Part model, mm, in its own coordinate system. Round coordinates to 2 decimals unless told otherwise and drop trailing zeros. Loops run counter-clockwise (first coordinate to the right, second up) from the corner with the lowest first, then second, coordinate; pieces in that order, holes last. Notation, with made-up numbers: (50, 82.5) -> (77, 82.5) arc R16 ccw to (77, 97.5) -> close; hole circle Ø1 at (31, 54.25). An arc over 180 degrees is marked (long way). Use a Markdown table: item, result. Add a question column.
Item 1: Cut at D-D, the plane x = -18. List the corners of the cut face in (y, z).
Item 2: Flat gauge pins, fed straight in: pin 1 (1.2 mm diameter, centred on y = 4.5, z = 1.5, fed in from -X); pin 2 (0.7 mm diameter, centred on y = 31, z = 1, fed in from -X); pin 3 (1.2 mm diameter, centred on x = -16.5, z = 1.5, fed in from -Y). Where does each tip first touch, or does it go through?
Item 3: Cut at B-B, the plane z = 1.8. List the corners of the cut face in (x, y).
Item 4: Cut at A-A, the plane x = -11.65. List the corners of the cut face in (y, z), plus the area to 3 significant figures.
Item 5: Probe line 1 (Y direction, x = -14.75, z = 0.55); line 2 (Y direction, x = -12.25, z = 1.5); line 3 (X direction, y = 31, z = 2.05). List the from-to ranges inside material, lowest first. Write a range as [from, to].
Item 6: Cut at C-C, the plane y = 50.5. List the corners of the cut face in (x, z), plus the area to 4 significant figures.
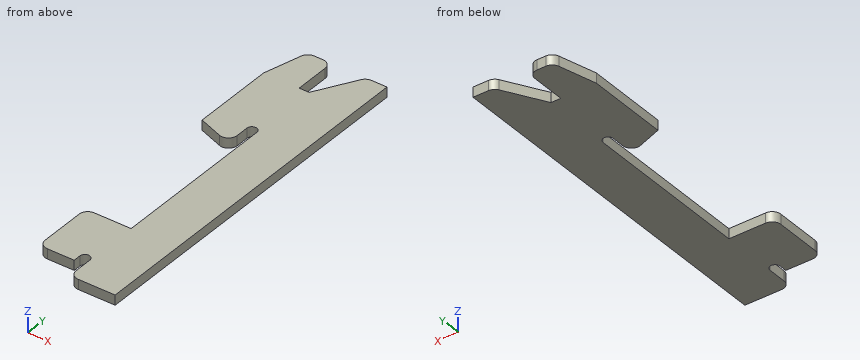
```python
from build123d import *

# Parameters (mm, degrees)
F1_DEPTH = 2.3


with BuildPart() as f1:
    # F0 (on Top) → F1 (new body)
    with BuildSketch(Plane.XY):
        with BuildLine():
            Line((-8.5, 0), (0, 0))
            Line((0, 0), (0, 84))
            Line((0, 84), (-3.571797, 84))
            ThreePointArc((-3.571797, 84), (-4.571797, 83.732051), (-5.303848, 83))
            Line((-5.303848, 83), (-10.5, 74))
            Line((-10.5, 74), (-12.8, 74))
            Line((-12.8, 74), (-12.8, 82))
            ThreePointArc((-12.8, 82), (-13.385786, 83.414214), (-14.8, 84))
            Line((-14.8, 84), (-16.785854, 84))
            ThreePointArc((-16.785854, 84), (-18.003377, 83.586707), (-18.717706, 82.517638))
            Line((-18.717706, 82.517638), (-21, 74))
            Line((-21, 74), (-21, 54.984556))
            Line((-21, 54.984556), (-15.48404, 52.976911))
            ThreePointArc((-15.48404, 52.976911), (-13.652847, 53.217992), (-12.8, 54.856296))
            Line((-12.8, 54.856296), (-12.8, 57.85))
            ThreePointArc((-12.8, 57.85), (-11.65, 59), (-10.5, 57.85))
            Line((-10.5, 57.85), (-10.5, 19))
            Line((-10.5, 19), (-19, 19))
            ThreePointArc((-19, 19), (-20.414214, 18.414214), (-21, 17))
            Line((-21, 17), (-21, 6.5))
            ThreePointArc((-21, 6.5), (-20.414214, 5.085786), (-19, 4.5))
            Line((-19, 4.5), (-12.8, 4.5))
            Line((-12.8, 4.5), (-12.8, 6.25))
            ThreePointArc((-12.8, 6.25), (-11.65, 7.4), (-10.5, 6.25))
            Line((-10.5, 6.25), (-10.5, 2))
            ThreePointArc((-10.5, 2), (-9.914214, 0.585786), (-8.5, 0))
        make_face()
    extrude(amount=F1_DEPTH)


solid = f1.part
```
A:
| question | item | result |
|---|---|---|
| 1 | outline | (4.5, 0) -> (19, 0) -> (19, 2.3) -> (4.5, 2.3) -> close; (53.89, 0) -> (83.59, 0) -> (83.59, 2.3) -> (53.89, 2.3) -> close |
| 2 | pin 1 | stops at x = -20.43 |
| 2 | pin 2 | stops at x = -10.5 |
| 2 | pin 3 | stops at y = 4.5 |
| 3 | outline | (-21, 6.5) arc R2 ccw to (-19, 4.5) -> (-12.8, 4.5) -> (-12.8, 6.25) arc R1.15 cw to (-10.5, 6.25) -> (-10.5, 2) arc R2 ccw to (-8.5, 0) -> (0, 0) -> (0, 84) -> (-3.57, 84) arc R2 ccw to (-5.3, 83) -> (-10.5, 74) -> (-12.8, 74) -> (-12.8, 82) arc R2 ccw to (-14.8, 84) -> (-16.79, 84) arc R2 ccw to (-18.72, 82.52) -> (-21, 74) -> (-21, 54.98) -> (-15.48, 52.98) arc R2 ccw to (-12.8, 54.86) -> (-12.8, 57.85) arc R1.15 cw to (-10.5, 57.85) -> (-10.5, 19) -> (-19, 19) arc R2 ccw to (-21, 17) -> close |
| 4 | outline | (7.4, 0) -> (19, 0) -> (19, 2.3) -> (7.4, 2.3) -> close; (59, 0) -> (74, 0) -> (74, 2.3) -> (59, 2.3) -> close |
| 4 | area | 61.2 mm^2 |
| 5 | line 1 | y = [4.5, 19], [52.86, 84] |
| 5 | line 2 | y = [7.23, 19], [58.83, 74] |
| 5 | line 3 | x = [-10.5, 0] |
| 6 | outline | (-10.5, 0) -> (0, 0) -> (0, 2.3) -> (-10.5, 2.3) -> close |
| 6 | area | 24.15 mm^2 |
